Source: three-view drawing plus pictorial views. Frame: mm from the lowest corner of the part. Coordinates: 2 decimals unless noted, no trailing zeros. Loops run counter-clockwise (first coordinate to the right, second up) from the corner with the lowest first, then second, coordinate; pieces in that order, holes last.
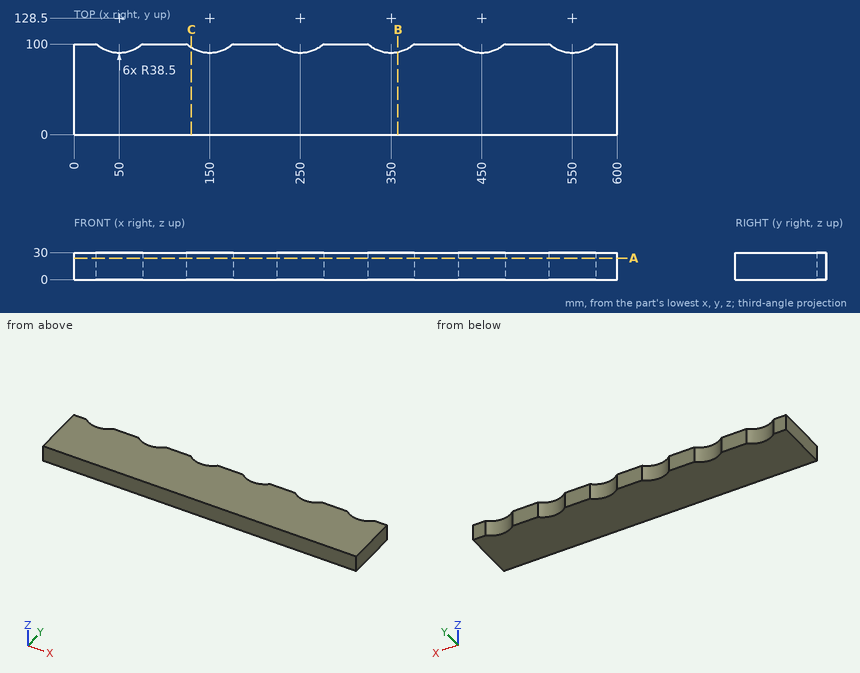
Q1. Line query: line 1 along Y through (x, z) = (344, 24); line 2 along Y through (x, z) = (525, 24). Output: solid intervals per line, ascending.
Q2. Section B-B, the plane x = 357.5. Return the cut outline in (y, z), plus the area to 3 significant figures.
Q3. Section C-C, the plane x = 129.5. Return the cut outline in (y, z), plus the area to 3 significant figures.
Q4. Section A-A, the plane z = 23.75. Return the cut outline in (x, y).
Q5. Contact query for flat-ended pins moving along their axis: pin 1 Ø1.5 at (x, z) = (151, 11.5) entering from +Y; pin 2 Ø5 at (x, z) = (351, 7.5) entering from +Y. Output: stop coordinate, or through.
Derived:
1. line 1: y = 0 to 90.47
1. line 2: y = 0 to 99.22
2. outline: (0, 0) - (90.74, 0) - (90.74, 30) - (0, 30) - close
2. area: 2,720 mm2
3. outline: (0, 0) - (95.91, 0) - (95.91, 30) - (0, 30) - close
3. area: 2,880 mm2
4. outline: (0, 0) - (600, 0) - (600, 100) - (575.88, 100) arc R38.5 cw to (524.12, 100) - (475.88, 100) arc R38.5 cw to (424.12, 100) - (375.88, 100) arc R38.5 cw to (324.12, 100) - (275.88, 100) arc R38.5 cw to (224.12, 100) - (175.88, 100) arc R38.5 cw to (124.12, 100) - (75.88, 100) arc R38.5 cw to (24.12, 100) - (0, 100) - close
5. pin 1: stops at y = 90.04
5. pin 2: stops at y = 90.16
